Part model, mm, in its own coordinate system. A direction names the side the tool comes from. Round coordinates to 2 decimals unless told otherwise and drop trailing zeros. Order: outer loops, then holes, each group sorted by start corner. A loop starts at its lowest first (then second) coordinate and runs counter-clockwise, first axis right, second up. Notation, with made-up numbers: (14, 75) -> (38, 75) arc R26 cw to (38, 104) -> close; hole circle Ø1 at (74.5, 1.5). An arc over 180 degrees is marked (long way). Return JSON: item names as keys, results as strings. Group by question number.
Autodesk Inventor part; units mm, degrees
ref_plane "Start plane" through (0, 0, 10.2219) normal (0, 0, 1) x (1, 0, 0)
ref_plane "End plane" through (0, 0, 785.2713) normal (0, 0, 1) x (1, 0, 0)
ref_plane "Work Plane4" through (344.6079, 0, 575.4319) normal (0.4912, 0, 0.871) x (0.871, 0, -0.4912)
ref_plane "Start plane" through (0, 0, 10.2219) normal (0, 0, 1) x (1, 0, 0)
ref_plane "End plane" through (0, 0, 785.2713) normal (0, 0, 1) x (1, 0, 0)
sketch "Sketch" plane through (0, 0, 0) normal (0, 0, 1) x (1, 0, 0)
  line L0 (-17.5, -14.3) -> (-17.5, 14.3)
  line L1 (-14.3, 17.5) -> (14.3, 17.5)
  line L2 (17.5, 14.3) -> (17.5, -14.3)
  line L3 (14.3, -17.5) -> (-14.3, -17.5)
  arc A0 (-17.5, -14.3) -> (-14.3, -17.5) centre (-14.3, -14.3) ccw
  arc A1 (-14.3, 17.5) -> (-17.5, 14.3) centre (-14.3, 14.3) ccw
  arc A2 (17.5, 14.3) -> (14.3, 17.5) centre (14.3, 14.3) ccw
  arc A3 (14.3, -17.5) -> (17.5, -14.3) centre (14.3, -14.3) ccw
  arc A4 (-14.3, 15.9) -> (-15.9, 14.3) centre (-14.3, 14.3) ccw
  line L4 (-14.3, 15.9) -> (14.3, 15.9)
  arc A5 (15.9, 14.3) -> (14.3, 15.9) centre (14.3, 14.3) ccw
  line L5 (15.9, 14.3) -> (15.9, -14.3)
  arc A6 (14.3, -15.9) -> (15.9, -14.3) centre (14.3, -14.3) ccw
  line L6 (14.3, -15.9) -> (-14.3, -15.9)
  arc A7 (-15.9, -14.3) -> (-14.3, -15.9) centre (-14.3, -14.3) ccw
  line L7 (-15.9, -14.3) -> (-15.9, 14.3)
  line L8 (0, 25.4278) -> (0, -25.4278) construction
  line L9 (-25.4278, 0) -> (25.4278, 0) construction
  dimension "d7" = 3.2
  dimension "d10" = 35
  dimension "d11" = 35
  dimension "d12" = 1.6
  dimension "d15" = 17.5
  dimension "d16" = 17.5
extrude "Body" add sketch "Sketch" along normal up to surface (775.0495 mm away) from surface at 10.2219
sketch "Sketch3" plane through (0, 0, 0) normal (0, 0, 1) x (1, 0, 0)
  line L0 (0, 0) -> (10, 0)
ref_plane "Work Plane3" through (0, 0, 0) normal (0, -1, 0) x (1, 0, 0)
sketch "Sketch4" plane through (0, 0, 0) normal (0, -1, 0) x (1, 0, 0)
  line L0 (-2, 10.2219) -> (12, 10.2219)
  line L1 (-2, 785.2713) -> (12, 785.2713)
  dimension "d18" = 775.0495
ref_plane "Work Plane4" through (344.6079, 0, 575.4319) normal (0.4912, 0, 0.871) x (0.871, 0, -0.4912)
split "Split1" plane through (344.6079, 0, 575.4319) removes the side toward (0.4912, 0, 0.871)
ref_plane "Work Plane5" through (-331.3145, 0, 166.7549) normal (-0.871, 0, 0.4912) x (0.4912, 0, 0.871)
split "Split2" plane through (-331.3145, 0, 166.7549) removes the side toward (-0.871, 0, 0.4912)
ref_plane "Work Plane6" through (-23.8395, 0, -6.6467) normal (0.871, 0, -0.4912) x (-0.4912, 0, -0.871)
split "Split3" plane through (-23.8395, 0, -6.6467) removes the side toward (0.871, 0, -0.4912)
ref_plane "Work Plane7" through (-344.6079, 0, 214.4339) normal (-0.4912, 0, -0.871) x (-0.871, 0, 0.4912)
split "Split4" plane through (-344.6079, 0, 214.4339) removes the side toward (-0.4912, 0, -0.871)
equation "\"d7\" = G_IR"
equation "\"d10\" = G_H"
equation "\"d11\" = G_W"
equation "\"d12\" = G_T"
equation "\"d15\" = 0.5 * d10"
equation "\"d16\" = 0.5 * d11"
equation "\"d3\" = G_L"
equation "\"G_W\" = 35"
equation "\"G_H\" = 35"
equation "\"G_T\" = 1.6"
equation "\"G_IR\" = 3.2"
equation "\"G_L\" = d18"
equation "\"G_OFFSET_START\" = -10.22188"
equation "\"G_OFFSET_END\" = -4.59446"
equation "\"d13\" = -G_OFFSET_START"
equation "\"d14\" = G_OFFSET_END + B_L"
equation "\"B_L\" = 789.86581"
properties part number "AS 1163 - C350L0 35x35x1.6 SHS - 775.049" material "Steel, Mild"
(1) Probe L1, parallel to Y at x = 7, z = 449; L2, parallel to X at y = 5, z = 730.5. List the from-to ranges inside material, lowest first. Write a range as [from, to].
(2) Mould opens along X. For faces 1 (the flat face through (17.5, 0, 408)), 2 (the flat face through (0, -17.5, 390)), 3 (the flat face through (0, -15.9, 390)), 4 (the flat face through (-17.5, 0, 372)) say: pulls with the +X half, pulls with the -X half, needs draft (parallel to the pull), parting line crosses it, or undercut.
(3) Saw through at B-B, the plane z = 150. List the corners of the cut face in (x, y), and give its area (3 significant figures).
(4) Saw through at A-A, the plane y = -2. List the corners of the cut face in (x, z), and give its area (3 significant figures).
(5) Tool access for faces 5 (the flat face through (-16.215, -1.378, 725.492)), 6 (the flat face through (0, 15.9, 390)): list every direction of +Z, -Z, +X, -X, +Y, -Y with a clear straight run to the whole face (end or side of a thin tool).
(6) Saw through at C-C, the plane x = 1. List the corners of the cut face in (y, z), and give its area (3 significant figures).
(7) Pin check, flat tip, straight feed: P1, Ø4, axis at x = -13.5, y = 13, coming from the -Z side. Stop position of the tip, or through.
Results are:
{
 "1": {"L1": "y = [-17.5, -15.9], [15.9, 17.5]", "L2": "x = [15.9, 17.5]"},
 "2": {"face 1": "pulls with the +X half", "face 2": "needs draft", "face 3": "undercut", "face 4": "pulls with the -X half"},
 "3": {"outline": "(-17.5, -14.3) arc R3.2 ccw to (-14.3, -17.5) -> (14.3, -17.5) arc R3.2 ccw to (17.5, -14.3) -> (17.5, 14.3) arc R3.2 ccw to (14.3, 17.5) -> (-14.3, 17.5) arc R3.2 ccw to (-17.5, 14.3) -> close; hole (-15.9, -14.3) arc R1.6 ccw to (-14.3, -15.9) -> (14.3, -15.9) arc R1.6 ccw to (15.9, -14.3) -> (15.9, 14.3) arc R1.6 ccw to (14.3, 15.9) -> (-14.3, 15.9) arc R1.6 ccw to (-15.9, 14.3) -> close", "area": "207 mm^2"},
 "4": {"outline": "(-17.5, 29.96) -> (-15.9, 29.06) -> (-15.9, 726.05) -> (-17.5, 723.21) -> close; (15.9, 63.82) -> (17.5, 66.66) -> (17.5, 759.9) -> (15.9, 760.81) -> close", "area": "2,220 mm^2"},
 "5": {"face 5": "+Z, -X, +Y, -Y", "face 6": "+Z, -Z"},
 "6": {"outline": "(-17.5, 37.4) -> (-15.9, 37.4) -> (-15.9, 756.02) -> (-17.5, 756.02) -> close; (15.9, 37.4) -> (17.5, 37.4) -> (17.5, 756.02) -> (15.9, 756.02) -> close", "area": "2,300 mm^2"},
 "7": {"P1": "passes through"}
}
